from build123d import *

# Parameters (mm, degrees)
SKETCH_W        = 76
SKETCH_H        = 22
PAD_DEPTH       = 76
SKETCH001_W     = 66
SKETCH001_H     = 26
PAD001_DEPTH    = 47
SKETCH002_W     = 62
SKETCH002_H     = 22
POCKET_DEPTH    = 45
SKETCH003_W     = 72
SKETCH003_H     = 18
POCKET001_DEPTH = 74
SKETCH004_W     = 30
SKETCH004_H     = 2
POCKET002_DEPTH = 45
SKETCH005_W     = 30
SKETCH005_H     = 2
POCKET003_DEPTH = 74
SKETCH006_W     = 26
SKETCH006_H     = 2
POCKET004_DEPTH = 15
FILLET_R        = 10
FILLET001_R     = 10
FILLET002_R     = 2
FILLET003_R     = 2
FILLET004_R     = 2
FILLET005_R     = 2


with BuildPart() as part:
    # Sketch → Pad (new body)
    with BuildSketch(Plane.XY):
        with Locations((38, 11)):
            Rectangle(SKETCH_W, SKETCH_H)
    extrude(amount=PAD_DEPTH)

    # Sketch001 → Pad001 (join)
    with BuildSketch(Plane.XY):
        with Locations((38, -13)):
            Rectangle(SKETCH001_W, SKETCH001_H)
    extrude(amount=PAD001_DEPTH)

    # Sketch002 (on Face4 of Pad001) → Pocket (cut)
    with BuildSketch(Plane.XY.offset(47)):
        with Locations((38, -13)):
            Rectangle(SKETCH002_W, SKETCH002_H)
    extrude(amount=-POCKET_DEPTH, mode=Mode.SUBTRACT)

    # Sketch003 (on Face7 of Pocket) → Pocket001 (cut)
    with BuildSketch(Plane.XY.offset(76)):
        with Locations((38, 11)):
            Rectangle(SKETCH003_W, SKETCH003_H)
    extrude(amount=-POCKET001_DEPTH, mode=Mode.SUBTRACT)

    # Sketch004 (on Face4 of Pocket001) → Pocket002 (cut)
    with BuildSketch(Plane.XY.offset(47)):
        with Locations((38, -1)):
            Rectangle(SKETCH004_W, SKETCH004_H)
    extrude(amount=-POCKET002_DEPTH, mode=Mode.SUBTRACT)

    # Sketch005 (on Face8 of Pocket002) → Pocket003 (cut)
    with BuildSketch(Plane.XY.offset(76)):
        with Locations((38, 1)):
            Rectangle(SKETCH005_W, SKETCH005_H)
    extrude(amount=-POCKET003_DEPTH, mode=Mode.SUBTRACT)

    # Sketch006 (on Face4 of Pocket003) → Pocket004 (cut)
    with BuildSketch(Plane.XY.offset(47)):
        with Locations((38, -25)):
            Rectangle(SKETCH006_W, SKETCH006_H)
    extrude(amount=-POCKET004_DEPTH, mode=Mode.SUBTRACT)

    # Fillet
    fillet_edges = [part.edges().sort_by_distance(p)[0] for p in [
        (51, -25, 47),
    ]]
    fillet(fillet_edges, radius=FILLET_R)

    # Fillet001
    fillet001_edges = [part.edges().sort_by_distance(p)[0] for p in [
        (25, -25, 47),
    ]]
    fillet(fillet001_edges, radius=FILLET001_R)

    # Fillet002
    fillet002_edges = [part.edges().sort_by_distance(p)[0] for p in [
        (5, -26, 23.5),
    ]]
    fillet(fillet002_edges, radius=FILLET002_R)

    # Fillet003
    fillet003_edges = [part.edges().sort_by_distance(p)[0] for p in [
        (71, -26, 23.5),
    ]]
    fillet(fillet003_edges, radius=FILLET003_R)

    # Fillet004
    fillet004_edges = [part.edges().sort_by_distance(p)[0] for p in [
        (76, 0, 38),
    ]]
    fillet(fillet004_edges, radius=FILLET004_R)

    # Fillet005
    fillet005_edges = [part.edges().sort_by_distance(p)[0] for p in [
        (0, 0, 38),
    ]]
    fillet(fillet005_edges, radius=FILLET005_R)


solid = part.part
Work out the finished part from the listing and answer in its coordinate system (mm). A direction names the side the tool comes from. Give positions to 0.01 mm unless a question says otherwise; leave off trailing zeros. Write each loop counter-clockwise with the first axis right and the second up, starting at its lowest first coordinate (ties: lowest second). Pieces come first, ordered by that corner, then holes. Notation, with made-up numbers: (28, -36) - (62, -36) arc R36 cw to (62, 2) - close; hole circle Ø11 at (61.25, -22). An arc over 180 degrees is marked (long way). One line per item, written item: value. Start each with the question number.
1. Consider probe 1 along Y at (x, z) = (20, 8.5); probe 2 along X at (y, z) = (7.5, 68); probe 3 along Y at (x, z) = (58.5, 72). Determine where each line is inside the solid, lowest interval first.
2. Find section A-A (z = 7). Write down the section's boundary in (x, y).
3. For a pull along X with two mould halves and no side action, classify faces 6 (the cylindrical face through (70.4, -25.43, 23.83)), 7 (the cylindrical face through (5.6, -25.43, 23.83)), 8 (the flat face through (66, 0, 54)), 9 (the flat face through (51, -25, 35)) as +X half, -X half, draft (parallel to the pull), parting line (faces both ways), or undercut.
4. Given pin 1 (1 mm diameter, centred on x = 35, y = -25, fed in from +Z); pin 2 (1.6 mm diameter, centred on y = -25, z = 34.5, fed in from +X); pin 3 (1.5 mm diameter, centred on x = 47.5, z = 46, fed in from -Y); pin 4 (8 mm diameter, centred on y = -2, z = 48.5, fed in from +X), each flat-ended and moving along its own axis, determine where each tip first touches the part or whether it passes through.
5. For faces 1 (the flat face through (69.3, -10.1, 47)), 2 (the cylindrical face through (54.01, -24.99, 44.15)), 3 (the flat face through (23, 0, 31)), 4 (the flat face through (38, -26, 23)), 5 (the flat face through (38, 21, 76)), determine the directions among +Z, -Z, +X, -X, +Y, -Y from which every point of the face is accessible in a straight line to the end or side of a thin tool.
6. Find section D-D (z = 68.5). Write down the section's boundary in (x, y), then the cut area to 3 significant figures.
7. Find section C-C (y = -1). Write down the section's boundary in (x, z).
8. Find section B-B (x = 46). Write down the section's boundary in (y, z), then the cut area to 3 significant figures.
Geometry results:
1. probe 1: -26 to -24, -2 to 2, 20 to 22
1. probe 2: 0 to 2, 74 to 76
1. probe 3: 0 to 2, 20 to 22
2. outline: (0, 2) arc R2 ccw to (2, 0) - (5, 0) - (5, -24) arc R2 ccw to (7, -26) - (69, -26) arc R2 ccw to (71, -24) - (71, 0) - (74, 0) arc R2 ccw to (76, 2) - (76, 22) - (0, 22) - close; hole (2, 2) - (23, 2) - (23, -2) - (7, -2) - (7, -24) - (69, -24) - (69, -2) - (53, -2) - (53, 2) - (74, 2) - (74, 20) - (2, 20) - close
3. face 6: +X half
3. face 7: -X half
3. face 8: draft
3. face 9: undercut
4. pin 1: z = 32
4. pin 2: x = 70.99
4. pin 3: y = 20
4. pin 4: x = 76
5. face 1: +Z, +X, -X, -Y
5. face 2: +Z, -Y
5. face 3: +Z
5. face 4: +Z, -Z, +X, -X, -Y
5. face 5: +Z, +X, -X, +Y, -Y
6. outline: (0, 2) arc R2 ccw to (2, 0) - (23, 0) - (23, 2) - (2, 2) - (2, 20) - (74, 20) - (74, 2) - (53, 2) - (53, 0) - (74, 0) arc R2 ccw to (76, 2) - (76, 22) - (0, 22) - close
6. area: 314 mm2
7. outline: (5, 0) - (71, 0) - (71, 47) - (53, 47) - (53, 2) - (23, 2) - (23, 47) - (5, 47) - close
8. outline: (-26, 0) - (22, 0) - (22, 76) - (20, 76) - (20, 2) - (-24, 2) - (-24, 32) - (-26, 32) - close
8. area: 304 mm2
